Geometry: final body of the model. Coordinates: model frame, mm. Give positions to 0.01 mm unless a question says otherwise; leave off trailing zeros. Write each loop counter-clockwise with the first axis right and the second up, starting at its lowest first coordinate (ties: lowest second). Pieces come first, ordered by that corner, then holes. Notation, with made-up numbers: (84, -22.75) - (105, -22.75) arc R16 ccw to (105, -0.75) - close; hole circle Ø4 at (65.25, 19). An arc over 180 degrees is marked (long way). Return JSON: item names as keys, results as strings.
from build123d import *

# Parameters (mm, degrees)
SKETCH1_R           = 1.55
SKETCH1_R_2         = 1.5
BOSS_EXTRUDE1_DEPTH = 4


with BuildPart() as part:
    # Sketch1 → Boss-Extrude1 (new body)
    with BuildSketch(Plane.XY):
        with BuildLine():
            Line((-18, -2.263569898), (18, -2.263569898))
            ThreePointArc((18, -2.263569898), (19.414213562, -1.677783461), (20, -0.263569898))
            Line((20, -0.263569898), (20, 0.263569898))
            ThreePointArc((20, 0.263569898), (19.414213562, 1.677783461), (18, 2.263569898))
            Line((18, 2.263569898), (-18, 2.263569898))
            ThreePointArc((-18, 2.263569898), (-19.414213562, 1.677783461), (-20, 0.263569898))
            Line((-20, 0.263569898), (-20, -0.263569898))
            ThreePointArc((-20, -0.263569898), (-19.414213562, -1.677783461), (-18, -2.263569898))
        make_face()
        Circle(SKETCH1_R, mode=Mode.SUBTRACT)
        with Locations((-17, 0)):
            Circle(SKETCH1_R_2, mode=Mode.SUBTRACT)
        with Locations(Location((17, 0, 0), (0, 0, 180))):
            Circle(SKETCH1_R_2, mode=Mode.SUBTRACT)
    extrude(amount=BOSS_EXTRUDE1_DEPTH)


solid = part.part
Q1. Section query A-A, the plane x = 17. Return the cut outline in (y, z).
Answer key:
{"outline": "(-2.26, 0) - (-1.5, 0) - (-1.5, 4) - (-2.26, 4) - close; (1.5, 0) - (2.26, 0) - (2.26, 4) - (1.5, 4) - close"}
Q2. Section query C-C, the plane x = 0. Return the cut outline in (y, z), plus the area to 3 significant figures.
Answer key:
{"outline": "(-2.26, 0) - (-1.55, 0) - (-1.55, 4) - (-2.26, 4) - close; (1.55, 0) - (2.26, 0) - (2.26, 4) - (1.55, 4) - close", "area": "5.71 mm^2"}
Q3. Section query B-B, the plane z = 2.35. Return the cut outline in (x, y), plus the area to 3 significant figures.
Answer key:
{"outline": "(-20, -0.26) arc R2 ccw to (-18, -2.26) - (18, -2.26) arc R2 ccw to (20, -0.26) - (20, 0.26) arc R2 ccw to (18, 2.26) - (-18, 2.26) arc R2 ccw to (-20, 0.26) - close; hole circle Ø3 at (-17, 0); hole circle Ø3.1 at (0, 0); hole circle Ø3 at (17, 0)", "area": "156 mm^2"}
Q4. Material intervals for probe 1 along Y at (x, z) = (0, 2.3); probe 2 along X at (y, z) = (-0.75, 2.45); probe 3 along X at (y, z) = (-1.35, 2.4), sorted ascending. Write a range as [from, to].
Answer key:
{"probe 1": "y = [-2.26, -1.55], [1.55, 2.26]", "probe 2": "x = [-19.94, -18.3], [-15.7, -1.36], [1.36, 15.7], [18.3, 19.94]", "probe 3": "x = [-19.68, -17.65], [-16.35, -0.76], [0.76, 16.35], [17.65, 19.68]"}
Q5. Pin query (flat end, axial travel): P1, Ø2.5, axis at x = -17, y = 0, coming from the -Z side. Return the tip coordinate at first contact, or that it passes through.
Answer key:
{"P1": "passes through"}
Q6. Section query D-D, the plane y = -1.9. Return the cut outline in (x, z), plus the area to 3 significant figures.
Answer key:
{"outline": "(-19.15, 0) - (19.15, 0) - (19.15, 4) - (-19.15, 4) - close", "area": "153 mm^2"}
Q7. Mould query, pull axis Y, two halves, no side actions, for faces 1 (the cylindrical face through (18.5, -0.07, 1.97)), 2 (the cylindrical face through (-19.43, -1.66, 1.97)), 3 (the cylindrical face through (-19.4, 1.69, 1.97)), 4 (the flat face through (0, 2, 0)). Classes: pulls with the +Y half, pulls with the -Y half, needs draft (parallel to the pull), parting line crosses it, or undercut.
Answer key:
{"face 1": "undercut", "face 2": "pulls with the -Y half", "face 3": "pulls with the +Y half", "face 4": "needs draft"}
